Geometry check sheet. Reference: the model listing, model coordinates, mm. A direction names the side the tool comes from. Coordinates: 2 decimals unless noted, no trailing zeros. Write each loop counter-clockwise with the first axis right and the second up, starting at its lowest first coordinate (ties: lowest second). Pieces come first, ordered by that corner, then holes. Notation, with made-up numbers: (20.5, 18) - (38.5, 18) arc R12 ccw to (38.5, 25) - close; hole circle Ø9 at (72.5, 27.25). An arc over 180 degrees is marked (long way). Answer as a JSON object with one key per item and string values. Group by question number.
from build123d import *

# Parameters (mm, degrees)
F1_DEPTH = 25
F2_W     = 4.965493
F2_H     = 6.25
F3_DEPTH = 12
F4_W     = 10
F4_H     = 20
F5_DEPTH = 10


with BuildPart() as f1:
    # F0 (on Top) → F1 (new body)
    with BuildSketch(Plane.XY):
        Polygon((110, -125), (110, 125), (-110, 125), (-110, -125), (-70, -125), (-49.67048, 65.990649), (50.32952, 65.990649), (70, -125), align=None)
    extrude(amount=F1_DEPTH)

    # F2 (on face) → F3 (cut)
    with BuildSketch(Plane(origin=(0, 125, 0), x_dir=(-1, 0, 0), z_dir=(0, 1, 0))):
        with Locations((92.517253, 21.875)):
            Rectangle(F2_W, F2_H)
    extrude(amount=-F3_DEPTH, mode=Mode.SUBTRACT)

    # F4 (on face) → F5 (cut)
    with BuildSketch(Plane(origin=(0, 0, 0), x_dir=(1, 0, 0), z_dir=(0, 0, -1))):
        with Locations((-90, 25)):
            Rectangle(F4_W, F4_H)
        with Locations((90, 25)):
            Rectangle(F4_W, F4_H)
    extrude(amount=-F5_DEPTH, mode=Mode.SUBTRACT)


solid = f1.part
(1) Section check C-C (z = 6). Record the cut outline in (x, y).
(2) Section check D-D (y = -24). Record the cut outline in (x, z), and give its area (3 significant figures).
(3) Draft check along X on faces 1 (the face through (-95, -25, 5)), 2 (the face through (-110, 2, 12)), 3 (the face through (110, -2, 12)), 4 (the face through (60.027, -28.168, 12.325)). Enter one of: +X half, -X half, draft (parallel to the pull), parting line (faces both ways), or undercut.
(4) Gauge pin test, flat end, axial feed: pin 1 (4 mm diameter, centred on x = -91.5, y = 120, fed in from +Z). Record the tip position at first contact, or that the pin passes through.
(5) Section check A-A (y = 35). Record the cut outline in (x, z), and give its area (3 significant figures).
(6) Set-up check for faces 5 (the face through (-95, 119, 22)), 6 (the face through (0, 65.991, 12)), 7 (the face through (-2, 85, 25)), 8 (the face through (90, -125, 12)), 9 (the face through (90, -15, 5)): record each of +Z, -Z, +X, -X, +Y, -Y from which the full face is reachable in a straight line by a thin tool's end or side.
(7) Material ranges on L1, parallel to Y at x = -88.5, z = 2.5; L2, parallel to X at y = -19, z = 6.5; L3, parallel to X at y = -37.5, z = 22.25, recorded low to high. Write a range as [from, to].
(8) Section check B-B (x = 92). Record the cut outline in (y, z).
Conclusion:
{
 "1": {"outline": "(-110, -125) - (-70, -125) - (-49.67, 65.99) - (50.33, 65.99) - (70, -125) - (110, -125) - (110, 125) - (-110, 125) - close; hole (-95, -35) - (-85, -35) - (-85, -15) - (-95, -15) - close; hole (85, -35) - (95, -35) - (95, -15) - (85, -15) - close"},
 "2": {"outline": "(-110, 0) - (-95, 0) - (-95, 10) - (-85, 10) - (-85, 0) - (-59.25, 0) - (-59.25, 25) - (-110, 25) - close; (59.6, 0) - (85, 0) - (85, 10) - (95, 10) - (95, 0) - (110, 0) - (110, 25) - (59.6, 25) - close", "area": "2,330 mm^2"},
 "3": {"face 1": "undercut", "face 2": "-X half", "face 3": "+X half", "face 4": "undercut"},
 "4": {"pin 1": "stops at z = 25"},
 "5": {"outline": "(-110, 0) - (-52.97, 0) - (-52.97, 25) - (-110, 25) - close; (53.52, 0) - (110, 0) - (110, 25) - (53.52, 25) - close", "area": "2,840 mm^2"},
 "6": {"face 5": "+Z, +Y", "face 6": "+Z, -Z, -Y", "face 7": "+Z, +X, -X, +Y, -Y", "face 8": "+Z, -Z, +X, -X, -Y", "face 9": "-Z"},
 "7": {"L1": "y = [-125, -35], [-15, 125]", "L2": "x = [-110, -95], [-85, -58.72], [59.08, 85], [95, 110]", "L3": "x = [-110, -60.69], [60.99, 110]"},
 "8": {"outline": "(-125, 0) - (-35, 0) - (-35, 10) - (-15, 10) - (-15, 0) - (125, 0) - (125, 25) - (-125, 25) - close"}
}
